from build123d import *

# Parameters (mm, degrees)
F0_R     = 2.5146
F1_DEPTH = 2.032
F2_R     = 4.0386
F2_R_2   = 2.5146
F3_DEPTH = 4.953
F5_DEPTH = 4.953


with BuildPart() as f1:
    # F0 (on Top) → F1 (new body)
    with BuildSketch(Plane.XY):
        with BuildLine():
            ThreePointArc((0.1932728669, -8.1129981936), (5.8063138645, -5.6696396179), (8.1153, 0))
            ThreePointArc((8.1153, 0), (4.7193819453, 6.6019336671), (-2.6262691705, 7.6785939035))
            ThreePointArc((-2.6262691705, 7.6785939035), (-7.243577354, 3.6590546875), (-7.7389628282, -2.4426519264))
            ThreePointArc((-7.7389628282, -2.4426519264), (-4.7193819453, -6.6019336671), (0.1932728669, -8.1129981936))
        make_face()
        Circle(F0_R, mode=Mode.SUBTRACT)
        with BuildLine():
            ThreePointArc((-2.6262691705, 7.6785939035), (4.7193819453, 6.6019336671), (8.1153, 0))
            Line((8.1153, 0), (10.1473, 0))
            ThreePointArc((10.1473, 0), (5.9010738252, 8.255), (-3.2838639549, 9.601246524))
            Line((-3.2838639549, 9.601246524), (-2.6262691705, 7.6785939035))
        make_face()
        with BuildLine():
            Line((0.241666699, -10.1444218414), (0.1932728669, -8.1129981936))
            ThreePointArc((0.1932728669, -8.1129981936), (-4.7193819453, -6.6019336671), (-7.7389628282, -2.4426519264))
            Line((-7.7389628282, -2.4426519264), (-9.6767312985, -3.0542705621))
            ThreePointArc((-9.6767312985, -3.0542705621), (-8.7465221148, -5.1445163217), (-7.3716789291, -6.9732379177))
            ThreePointArc((-7.3716789291, -6.9732379177), (-3.9017137862, -9.3671941808), (0.241666699, -10.1444218414))
        make_face()
        with BuildLine():
            ThreePointArc((-7.3716789291, -6.9732379177), (-8.7465221148, -5.1445163217), (-9.6767312985, -3.0542705621))
            Line((-9.6767312985, -3.0542705621), (-13.4904375036, -4.2579921738))
            ThreePointArc((-13.4904375036, -4.2579921738), (-15.3146238281, -9.0077325834), (-10.2769386502, -9.7214676552))
            Line((-10.2769386502, -9.7214676552), (-7.3716789291, -6.9732379177))
        make_face()
    extrude(amount=F1_DEPTH)

    # F2 (on face) → F3 (join)
    with BuildSketch(Plane.XY.offset(2.032)):
        with BuildLine():
            Line((-5.8403095484, -5.6346143141), (-7.3716789291, -6.9732379177))
            ThreePointArc((-7.3716789291, -6.9732379177), (-3.9017137862, -9.3671941808), (0.241666699, -10.1444218414))
            Line((0.241666699, -10.1444218414), (0.1932728669, -8.1129981936))
            ThreePointArc((0.1932728669, -8.1129981936), (-3.0834805795, -7.5066797991), (-5.8403095484, -5.6346143141))
        make_face()
        Circle(F2_R)
        Circle(F2_R_2, mode=Mode.SUBTRACT)
        with BuildLine():
            ThreePointArc((-2.6262691705, 7.6785939035), (4.7193819453, 6.6019336671), (8.1153, 0))
            Line((8.1153, 0), (10.1473, 0))
            ThreePointArc((10.1473, 0), (5.9010738252, 8.255), (-3.2838639549, 9.601246524))
            Line((-3.2838639549, 9.601246524), (-2.6262691705, 7.6785939035))
        make_face()
    extrude(amount=F3_DEPTH)

    # F4 (on face) → F5 (cut)
    with BuildSketch(Plane(origin=(0, 0, 0), x_dir=(1, 0, 0), z_dir=(0, 0, -1))):
        with BuildLine():
            ThreePointArc((-3.0752344649, 7.5100617225), (-1.4721782365, 7.9806506834), (0.1932728669, 8.1129981936))
            Line((0.1932728669, 8.1129981936), (0.241666699, 10.1444218414))
            ThreePointArc((0.241666699, 10.1444218414), (-0.4196244465, 10.1386198574), (-1.079133301, 10.0897556268))
            Line((-1.079133301, 10.0897556268), (-3.0752344649, 7.5100617225))
        make_face()
        with BuildLine():
            ThreePointArc((7.9651252816, -6.2868494923), (9.5862456953, -3.3274), (10.1473, 0))
            Line((10.1473, 0), (8.1153, 0))
            ThreePointArc((8.1153, 0), (7.2163466693, -3.7124701802), (4.7186455722, -6.6024600002))
            Line((4.7186455722, -6.6024600002), (7.9651252816, -6.2868494923))
        make_face()
    extrude(amount=-F5_DEPTH, mode=Mode.SUBTRACT)


solid = f1.part
Input: part model. Units: mm. Frame: model coordinates. A direction names the side the tool comes from. Round coordinates to 2 decimals unless told otherwise and drop trailing zeros. Loops run counter-clockwise (first coordinate to the right, second up) from the corner with the lowest first, then second, coordinate; pieces in that order, holes last. Notation, with made-up numbers: M 17,51.25 L 66,51.25 A13 cw 66,61.25 Z; hole C -0.75,68 d5. An arc over 180 degrees is marked long. Answer as CSV lines item,"result". Start each with the question number.
(1) Line query: line 1 (Y direction, x = 0, z = 4); line 2 (X direction, y = 2, z = 5.25) (3 decimals); line 3 (Z direction, x = 0, y = -6.25). Output: solid intervals per line, ascending. Write a range as [from, to].
(2) Section D-D, the plane x = -14. Output: boundary loops of the cut face in (y, z), plus the area to 3 significant figures.
(3) Section C-C, the plane y = -1.75. Output: boundary loops of the cut face in (x, z) (3 decimals).
(4) Section A-A, the plane z = 2.75. Output: boundary loops of the cut face in (x, y).
(5) First-contact query: pin 1 (1.5 mm diameter, centred on y = -7.5, z = 6, fed in from +X); pin 2 (3 mm diameter, centred on x = -8.5, z = 2.5, fed in from -Y); pin 3 (1.5 mm diameter, centred on y = 3, z = 3, fed in from -X). Flat tips, straight axial feed; report the tip coordinate or a pass-through.
(6) Draft query along X for faces 4 (the cylindrical face through (-3.957, -9.344, 3.444)), 5 (the flat face through (-8.845, -8.367, 1.002)), 6 (the cylindrical face through (4.163, 9.254, 3.444)), 7 (the flat face through (8, 3, 4.953)). Return one class per face: released by +X, released by -X, zero draft, split by the parting line, or undercut.
(7) Reachability of faces 1 (the flat face through (-1, -9, 4.953)), 2 (the flat face through (-6.6, -6.3, 4.5)), 3 (the flat face through (-2.96, 8.65, 3.44)) from +Z, -Z, +X, -X, +Y, -Y: full face, straight path, thin tool, end or side. Return the list, or none.
(8) Section B-B, the plane y = 0.5. Output: boundary loops of the cut face in (x, z) (3 decimals), plus the area to 3 significant figures.
Values found:
1,line 1,"y = [-4.04, -2.51], [2.51, 4.04], [8.12, 10.15]"
1,line 2,"x = [-3.509, -1.524], [1.524, 3.509], [7.865, 9.948]"
1,line 3,"z = [0, 2.03]"
2,outline,"M -10.25,0 L -4.47,0 L -4.47,2.03 L -10.25,2.03 Z"
2,area,"11.8 mm²"
3,outline,"M -7.924,0 L -1.806,0 L -1.806,6.985 L -3.64,6.985 L -3.64,2.032 L -7.924,2.032 Z; M 1.806,0 L 7.924,0 L 7.924,2.032 L 3.64,2.032 L 3.64,6.985 L 1.806,6.985 Z"
4,outline,"M -7.37,-6.97 A10.15 ccw -1.08,-10.09 L -3.08,-7.51 A8.12 cw -5.84,-5.63 Z; C 0,0 d8.08; M -3.28,9.6 L -2.63,7.68 A8.12 cw 4.72,6.6 L 7.97,6.29 A10.15 ccw Z; hole C 0,0 d5.03"
5,pin 1,"stops at x = 0.2"
5,pin 2,"stops at y = -9.39"
5,pin 3,"stops at x = -3.35"
6,face 4,"undercut"
6,face 5,"undercut"
6,face 6,"split by the parting line"
6,face 7,"zero draft"
7,face 1,"-Z, +X"
7,face 2,"+Z, -X, +Y"
7,face 3,"+Z, -Z, -X"
8,outline,"M -8.1,0 L -2.464,0 L -2.464,6.985 L -4.008,6.985 L -4.008,2.032 L -8.1,2.032 Z; M 2.464,0 L 8.1,0 L 8.1,2.032 L 4.008,2.032 L 4.008,6.985 L 2.464,6.985 Z; M 8.1,4.953 L 10.135,4.953 L 10.135,6.985 L 8.1,6.985 Z"
8,area,"42.3 mm²"
